Part model, mm, in its own coordinate system. Face numbers are marked on the shaded views. A direction names the side the tool comes from. Give positions to 0.01 mm unless a question says otherwise; leave off trailing zeros. Order: outer loops, then holes, each group sorted by start corner. A loop starts at its lowest first (then second) coordinate and runs counter-clockwise, first axis right, second up. Notation, with made-up numbers: M 62.5,-38.5 L 110.5,-38.5 A31 cw 110.5,-1.5 Z; hole C 42.25,19 d8. An arc over 180 degrees is marked long. Return JSON: item names as keys, results as strings.
Autodesk Inventor part; units mm, degrees
ref_plane "YZ Plane" through (0, 0, 0) normal (1, 0, 0) x (0, 1, 0)
ref_plane "XZ Plane" through (0, 0, 0) normal (0, 1, 0) x (-1, 0, 0)
ref_plane "XY Plane" through (0, 0, 0) normal (0, 0, 1) x (1, 0, 0)
sketch "Sketch1" plane through (0, 0, 0) normal (1, 0, 0) x (0, 1, 0)
  line L0 (18.8, 0) -> (-18.8, 0)
  line L1 (-18.8, 0) -> (-18.8, 1.6)
  line L2 (-18.8, 1.6) -> (18.8, 1.6)
  line L3 (18.8, 1.6) -> (18.8, 0)
  line L4 (18.8, 1.6) -> (28.2, -7.7473)
  line L5 (28.2, -7.7473) -> (28.2, -20.4563)
  line L6 (28.2, -20.4563) -> (26.6, -20.4563)
  line L7 (26.6, -20.4563) -> (26.6, -7.7563)
  line L8 (26.6, -7.7563) -> (18.8, 0)
  line L9 (0, 0) -> (0, 1.6)
  line L10 (-18.8, 1.6) -> (-28.2, -7.7473)
  line L11 (-28.2, -7.7473) -> (-28.2, -20.4563)
  line L12 (-26.6, -20.4563) -> (-26.6, -7.7563)
  line L13 (-26.6, -7.7563) -> (-18.8, 0)
  line L14 (-28.2, -20.4563) -> (-26.6, -20.4563)
  dimension "d0" = 1.6
  dimension "d1" = 1.6
  dimension "d3" = 11
  dimension "d4" = 12.7
  dimension "d5" = 56.4
  dimension "d8" = 7.8
extrude "Extrusion1" add sketch "Sketch1" along normal blind 205.6
sketch "Sketch2" plane through (0, 28.2, -7.7473) normal (0, 1, 0) x (1, 0, 0)
  line L0 (0, 12.709) -> (0, 0)
  line L1 (0, 0) -> (205.6, 0)
  line L2 (205.6, 12.709) -> (205.6, 0)
  line L3 (0, 12.709) -> (205.6, 12.709)
  point P0 (0, -7.7473)
  point P1 (5.6, 6.3545)
  point P2 (200, 6.3545)
  point P3 (0, 6.3545)
  point P4 (205.6, 6.3545)
  dimension "d11" = 5.6
  dimension "d12" = 5.6
hole "Hole1" at (5.6, 28.2, -14.1018) at (200, 28.2, -14.1018) direction (0, -1, 0) diameter 2.459 end up to surface
sketch "Sketch3" plane through (0, -28.2, -20.4563) normal (0, -1, 0) x (1, 0, 0)
  circle A0 centre (200, 6.3545) radius 1.2295
  circle A1 centre (5.6, 6.3545) radius 1.2295
  point P0 (0, 20.4563)
hole "Hole2" at (200, -28.2, -14.1018) at (5.6, -28.2, -14.1018) direction (0, 1, 0) diameter 2.459 end up to surface
properties part number "ChassisMainBracket"
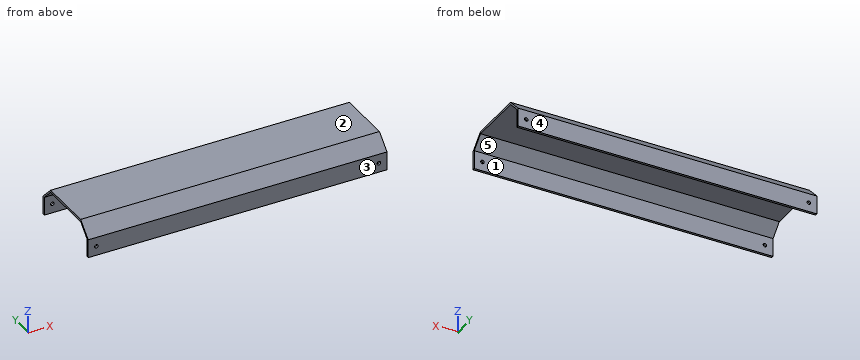
Q1. Band-saw the part on B-B (x = 30.5). Give the cut face in (y, z).
Established:
{"outline": "M -28.2,-20.46 L -26.6,-20.46 L -26.6,-7.76 L -18.8,0 L 18.8,0 L 26.6,-7.76 L 26.6,-20.46 L 28.2,-20.46 L 28.2,-7.75 L 18.8,1.6 L -18.8,1.6 L -28.2,-7.75 Z"}
Q2. Band-saw the part on C-C (y = 12). Give the cut face in (x, z), then the cut area to 3 significant figures.
Established:
{"outline": "M 0,0 L 205.6,0 L 205.6,1.6 L 0,1.6 Z", "area": "329 mm²"}
Q3. 3-axis set-ups, long thin cutter, end or side, ignore diameter. For the marked faces 4 and 5: which of +Z, -Z, +X, -X, +Y, -Y reach the whole face in a straight line?
Established:
{"face 4": "+Z, -Z, +X, -X, +Y", "face 5": "-Z, +X, -X"}
Q4. Probe line 1 along Y through (x, z) = (10, -14.75); line 2 along Z through (x, y) = (106.5, -11); line 3 along Z through (x, y) = (5.6, -27.4). List the from-to ranges inside material, lowest first.
Established:
{"line 1": "y = -28.2 to -26.6, 26.6 to 28.2", "line 2": "z = 0 to 1.6", "line 3": "z = -20.46 to -15.33, -12.87 to -6.95"}
Q5. Two-plate mould, pull along Y, no slides. Class the marked faces 1, 2 and 3: +Y half, -Y half, draft (parallel to the pull), parting line (faces both ways), or undercut.
Established:
{"face 1": "undercut", "face 2": "draft", "face 3": "-Y half"}
Q6. Band-saw the part on A-A (z = -18.5). Give the cut face in (x, y), then the cut area to 3 significant figures.
Established:
{"outline": "M 0,-28.2 L 205.6,-28.2 L 205.6,-26.6 L 0,-26.6 Z; M 0,26.6 L 205.6,26.6 L 205.6,28.2 L 0,28.2 Z", "area": "658 mm²"}
Q7. Pin check, flat tips, straight feed: pin 1 (12 mm diameter, centred on x = 112, y = -6.5, fed in from -Z); pin 2 (3 mm diameter, centred on x = 200, z = -14.1, fed in from +Y); pin 3 (6 mm diameter, centred on x = 39, y = 20, fed in from -Z). Stop position of each tip, or through.
Established:
{"pin 1": "stops at z = 0", "pin 2": "stops at y = 28.2", "pin 3": "stops at z = -4.18"}
